Input: part model. Units: mm. Frame: model coordinates. Face numbers are marked on the shaded views. A direction names the side the tool comes from. Give positions to 0.01 mm unless a question says otherwise; leave off trailing zeros. Loops run counter-clockwise (first coordinate to the right, second up) from the corner with the lowest first, then second, coordinate; pieces in that order, holes last. Notation, with made-up numbers: M 82,39.25 L 138,39.25 A37 ccw 138,77.25 Z; hole C 31,15 d3. An arc over 180 degrees is marked long. Use CSV: the item, a comma, the result in double quotes. Start each with the question number.
Q1. Pull-direction query (X, two-part tool) for the marked faces 3, 4 and 5; classes: released by +X, released by -X, zero draft, split by the parting line, or undercut.
Q2. Pin query (flat end, axial travel): pin 1 (0.8 mm diameter, centred on x = 0, y = -0.5, fed in from +Z). Return the tip coordinate at first contact, or that it passes through.
Q3. Reachability of the marked faces 1 and 2 from +Z, -Z, +X, -X, +Y, -Y: full face, straight path, thin tool, end or side. Return the list, or none.
Q4. Section A-A, the plane x = 0. Output: boundary loops of the cut face in (y, z) (3 decimals).
Q5. Material intervals for line 1 along Y through (x, z) = (0, 1.1) (3 decimals); line 2 along Y through (x, z) = (0.75, 0.9); line 3 along Z through (x, y) = (-1.25, 2.5), sorted ascending.
Q6. Section B-B, the plane z = 1.1. Output: boundary loops of the cut face in (x, y) (3 decimals), plus the area to 3 significant figures.
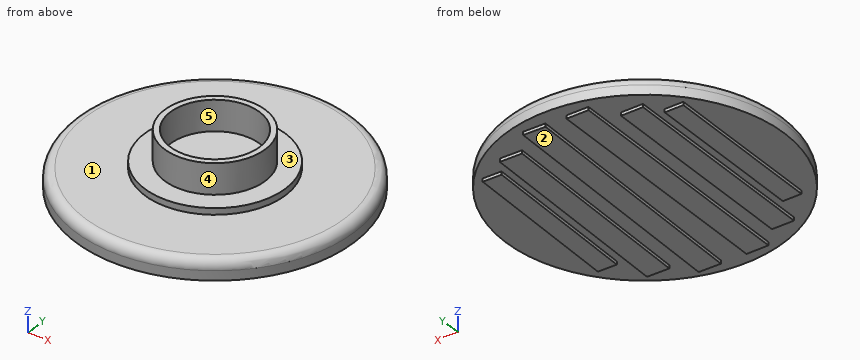
from build123d import *

# Parameters (mm, degrees)
F0_R     = 4.35
F1_DEPTH = 0.6
F2_R     = 2.2
F3_DEPTH = 0.2
F4_R     = 1.575
F4_R_2   = 1.395
F5_DEPTH = 0.95
F6_R     = 0.3
F7_W     = 0.580366
F7_H     = 5.113698
F7_W_2   = 0.687054
F7_H_2   = 6.536799
F7_W_3   = 0.685261
F7_H_3   = 7.790487
F8_DEPTH = 0.1


with BuildPart() as f1:
    # F0 (on Top) → F1 (new body)
    with BuildSketch(Plane.XY):
        Circle(F0_R)
    extrude(amount=F1_DEPTH)

    # F2 (on face) → F3 (join)
    with BuildSketch(Plane.XY.offset(0.6)):
        Circle(F2_R)
    extrude(amount=F3_DEPTH)

    # F4 (on face) → F5 (join)
    with BuildSketch(Plane.XY.offset(0.8)):
        Circle(F4_R)
        Circle(F4_R_2, mode=Mode.SUBTRACT)
    extrude(amount=F5_DEPTH)

    # F6
    f6_edges = [f1.edges().sort_by_distance(p)[0] for p in [
        (-4.35, 0, 0.6),
    ]]
    fillet(f6_edges, radius=F6_R)

    # F7 (on face) → F8 (join)
    with BuildSketch(Plane(origin=(0, 0, 0), x_dir=(1, 0, 0), z_dir=(0, 0, -1))):
        with Locations((-2.84447, -0.137814)):
            Rectangle(F7_W, F7_H)
        with Locations((-1.907698, 0.055486)):
            Rectangle(F7_W_2, F7_H_2)
        with Locations((-0.707726, -0.009958)):
            Rectangle(F7_W_3, F7_H_3)
        Polygon((1.110889, 3.865785), (0.42574, 3.878151), (0.285162, -3.911068), (0.970312, -3.923433), align=None)
        Polygon((1.496535, -3.24053), (2.183477, -3.252928), (2.301432, 3.282806), (1.61449, 3.295204), align=None)
        Polygon((3.168388, 2.362162), (2.588117, 2.372634), (2.495842, -2.740231), (3.076113, -2.750704), align=None)
    extrude(amount=F8_DEPTH)


solid = f1.part
A:
1,face 3,"zero draft"
1,face 4,"split by the parting line"
1,face 5,"undercut"
2,pin 1,"z = 0.8"
3,face 1,"+Z"
3,face 2,"-Z, +X, -X, +Y, -Y"
4,outline,"M -4.35,0 L 4.35,0 L 4.35,0.3 A0.3 ccw 4.05,0.6 L 2.2,0.6 L 2.2,0.8 L 1.575,0.8 L 1.575,1.75 L 1.395,1.75 L 1.395,0.8 L -1.395,0.8 L -1.395,1.75 L -1.575,1.75 L -1.575,0.8 L -2.2,0.8 L -2.2,0.6 L -4.05,0.6 A0.3 ccw -4.35,0.3 Z"
5,line 1,"-1.575 to -1.395, 1.395 to 1.575"
5,line 2,"-1.38 to -1.18, 1.18 to 1.38"
5,line 3,"0 to 0.6"
6,outline,"C 0,0 d3.15; hole C 0,0 d2.79"
6,area,"1.68 mm^2"
